Could you check a few things on this model? Use its own coordinates, in mm. Coordinates: 2 decimals unless noted, no trailing zeros. Loops run counter-clockwise (first coordinate to the right, second up) from the corner with the lowest first, then second, coordinate; pieces in that order, holes last.
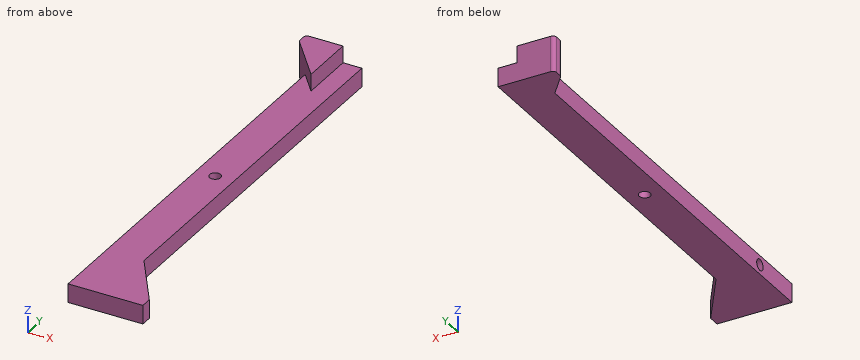
from build123d import *

# Parameters (mm, degrees)
F0_W      = 60
F0_H      = 10
F1_DEPTH  = 5
F4_DEPTH  = 5
F6_DEPTH  = 9.5
F8_D      = 3
F9_R      = 1
F11_D     = 3
F11_DEPTH = 4
F11_TIP   = 0.9012909285
F12_ANGLE = 90


with BuildPart() as f1:
    # F0 (on Right) → F1 (new body)
    with BuildSketch(Plane.YZ):
        with Locations((30, 10.0670714118)):
            Rectangle(F0_W, F0_H)
    extrude(amount=-F1_DEPTH)

    # F2: F1 across plane


with BuildPart() as f1_1:
    add(f1.part)
    add(f1.part.mirror(Plane.XZ))

    # F3 (on Right) → F4 (join)
    with BuildSketch(Plane.YZ):
        Polygon((-60, 25.0670714118), (-60, 15.0670714118), (-42, 15.0670714118), (-57, 25.0670714118), align=None)
    extrude(amount=-F4_DEPTH)

    # F5 (on face) → F6 (join)
    with BuildSketch(Plane.YZ):
        Polygon((60, 10), (45.0000320606, 10.031013164), (57, 0), (60, 0), align=None)
    extrude(amount=-F6_DEPTH)

    # F8 (through all)
    with Locations(Plane.YZ):
        with Locations((0, 10.122266598)):
            Hole(F8_D / 2)

    # F9
    f9_edges = [f1_1.edges().sort_by_distance(p)[0] for p in [
        (-4.75, 57, 0),
        (-4.75, 60, 0),
    ]]
    fillet(f9_edges, radius=F9_R)

    # F11
    with Locations(Plane(origin=(0, 0, 5.0670714118), x_dir=(1, 0, 0), z_dir=(0, 0, -1))):
        with Locations((-2.5, 45)):
            Hole(F11_D / 2, depth=F11_DEPTH)
            with Locations((0, 0, -(F11_DEPTH + F11_TIP / 2))):  # 118° drill point
                Cone(0, F11_D / 2, F11_TIP, mode=Mode.SUBTRACT)


with BuildPart() as f1_2:
    # F12: moved
    add(f1_1.part.rotate(Axis((-5, -4.5308351456, 5.0670714118), (0, 1, 0)), F12_ANGLE))


solid = f1_2.part
(1) For pin 1 (4 mm diameter, centred on y = 8.5, z = 2, fed in from +X); pin 2 (5.5 mm diameter, centred on y = 13.5, z = 2, fed in from -X); pin 3 (12 mm diameter, centred on x = 11.5, y = 26.5, fed in from +Z); pin 4 (2.5 mm diameter, centred on y = -45, z = 2.57, fed in from +X), each with a flat end and sliding along its axis, tell me the tip position at first contact or that it passes through.
Answers:
pin 1: stops at x = 5
pin 2: stops at x = -5
pin 3: passes through
pin 4: stops at x = 7.83
(2) Imagine slicing it at A-A, the plane y = 0. Write out the boundary of the cut face in (x, z).
Answers:
outline: (-5, 0.07) - (-1.44, 0.07) - (-1.44, 5.07) - (-5, 5.07) - close; (1.56, 0.07) - (5, 0.07) - (5, 5.07) - (1.56, 5.07) - close
(3) Imagine slicing it at D-D, the plane x = -3.5. Write out the boundary of the cut face in (y, z), and give its area (3 significant figures).
Answers:
outline: (-60, 0.07) - (60, 0.07) - (60, 9.57) - (49.14, 9.57) - (49.14, 5.07) - (-60, 5.07) - close; hole circle Ø3 at (-45, 2.57)
area: 642 mm2
(4) Imagine slicing it at C-C, the plane y = -18. Write out the boundary of the cut face in (x, z).
Answers:
outline: (-5, 0.07) - (5, 0.07) - (5, 5.07) - (-5, 5.07) - close
(5) I need wall thicknesses on probe 1 along Z at (x, y) = (-3.95, -45); probe 2 along X at (y, z) = (0, 2.1); probe 3 along X at (y, z) = (25, 1.75). Which ranges of each line are inside material? Lowest first, please.
Answers:
probe 1: z = 0.07 to 1.07, 4.07 to 5.07
probe 2: x = -5 to -1.44, 1.56 to 5
probe 3: x = -5 to 5
(6) Imagine slicing it at B-B, the plane x = 7. Write out the boundary of the cut face in (y, z).
Answers:
outline: (-60, 0.07) - (-45, 0.07) - (-45, 5.07) - (-60, 5.07) - close
